Could you check a few things on this model? Use its own coordinates, in mm. A direction names the side the tool comes from. Coordinates: 2 decimals unless noted, no trailing zeros. Loops run counter-clockwise (first coordinate to the right, second up) from the corner with the lowest first, then second, coordinate; pieces in that order, holes last.
1) Will these pins go through, and if not, where does the flat tip stop? P1, Ø8, axis at x = -11.5, z = 19, coming from the -Y side; P2, Ø2, axis at y = -26, z = 18, coming from the +X side; P3, Ø1.5, axis at y = 19, z = 15, coming from the -X side.
2) For faces 1 (the face through (-5.9, -37.15, 12.56)), 2 (the face through (4.52, -97.52, -4.35)), which set-ups out of +Z, -Z, +X, -X, +Y, -Y let a thin tool reach every point of the face, with its end or its side?
3) Imagine slicing it at A-A on y = -52. Please give me the cut outline in (x, z).
4) Thinking about a two-plate mould opening in Y: for faces 3 (the face through (-4.764, 5.484, 13.786)), 4 (the face through (-9.19, -104.525, 17.902)), 5 (the face through (-2, 83.25, 6.23)), 6 (the face through (1.7, -26.055, 0.225)), which applies, released by +Y, released by -Y, zero draft, split by the parting line, or undercut?
5) If I drill on line 1 along X through (y, z) = (19, 5.5); line 2 along Y through (x, z) = (-1, 5); line 3 along Z through (x, y) = (-7, -86), over which ranges is the centre line in solid material (lowest first)?
6) Imagine slicing it at B-B on z = 22. Please give me the cut outline in (x, y), plus the area to 3 significant figures.
Autodesk Inventor part; units mm, degrees
ref_plane "Work Plane2" through (0, -19.1092, 0) normal (0.8514, 0, 0.5245) x (0.513, -0.2079, -0.8328)
ref_plane "YZ Plane" through (0, 0, 0) normal (1, 0, 0) x (0, 1, 0)
ref_plane "XZ Plane" through (0, 0, 0) normal (0, 1, 0) x (-1, 0, 0)
ref_plane "Work Plane2" through (0, -19.1092, 0) normal (0.8514, 0, 0.5245) x (0.513, -0.2079, -0.8328)
ref_plane "Work Plane1" through (99.2081, 0, -373.4906) normal (0.8514, 0, 0.5245) x (0.513, -0.2079, -0.8328)
sketch "Sketch1" plane through (0, -19.1092, 0) normal (0.8514, 0, 0.5245) x (0.513, -0.2079, -0.8328)
  line L0 (-64.4031, -17.2568) -> (64.4031, 17.2568) construction
  line L1 (57.9081, 47.8134) -> (-73.8002, 26.9529) construction
  line L2 (-73.8887, 27.5118) -> (57.8196, 48.3724) construction
  line L3 (54.5542, 79.4406) -> (-78.6131, 72.4616) construction
  line L4 (-78.6427, 73.0267) -> (54.5245, 80.0057) construction
  line L5 (54.5245, 111.2451) -> (-78.6427, 118.2241) construction
  line L6 (64.5496, 16.7101) -> (-64.2566, -17.8034) construction
  line L7 (-50.2899, -60.7886) -> (74.2031, -13.0002) construction
  line L8 (-31.7037, -102.6067) -> (87.112, -42.0671) construction
  line L9 (74.4059, -13.5286) -> (-50.0871, -61.3169) construction
  line L10 (0.1465, -0.5466) -> (11.9566, -36.8944)
  line L11 (12.1594, -37.4227) -> (11.9566, -36.8944)
  line L12 (0, 0) -> (0.1465, -0.5466)
  line L13 (0, 0) -> (-7.946, 37.3832)
  line L14 (-8.0346, 37.9421) -> (-7.946, 37.3832)
  line L15 (12.1594, -37.4227) -> (27.7042, -72.3369)
  line L16 (-8.0346, 37.9421) -> (-12.0295, 75.9511)
  line L17 (-12.0591, 76.5162) -> (-12.0591, 114.7346)
  line L18 (-12.0591, 114.7346) -> (-51.1841, 106.4183)
  line L19 (-51.1841, 106.4183) -> (-11.4208, -80.6532)
  line L20 (-11.4208, -80.6532) -> (27.7042, -72.3369)
  line L21 (-12.0591, 76.5162) -> (-12.0295, 75.9511)
  line L22 (-5.7011, 18.3243) -> (-6.9685, 24.2871)
  line L23 (-5.7011, 18.3243) -> (-4.4336, 12.3615)
  line L24 (-6.9685, 24.2871) -> (-15.7828, 22.4135)
  line L25 (-13.2479, 10.488) -> (-4.4336, 12.3615)
  line L26 (-13.8552, 13.3451) -> (-15.1754, 19.5564)
  line L27 (-15.1754, 19.5564) -> (-15.7828, 22.4135)
  line L28 (-13.8552, 13.3451) -> (-13.2479, 10.488)
  line L29 (-23.1083, 11.3783) -> (-24.4286, 17.5896)
  line L30 (-24.4286, 17.5896) -> (-15.1754, 19.5564)
  line L31 (-13.8552, 13.3451) -> (-23.1083, 11.3783)
  line L32 (2.7351, -66.0118) -> (0.1524, -60.2107)
  line L33 (-12.2145, -27.9939) -> (-14.1768, -21.9547)
  line L34 (-29.827, 51.6736) -> (-30.4907, 57.9888)
  line L35 (-32.2968, 92.4504) -> (-32.2968, 98.8004)
  line L36 (-3.2177, -25.0707) -> (-5.1799, -19.0315)
  line L37 (11.3771, -62.1641) -> (8.7944, -56.3631)
  line L38 (-20.4189, 52.6624) -> (-21.0827, 58.9776)
  line L39 (-22.8369, 92.4504) -> (-22.8369, 98.8004)
  line L40 (2.7351, -66.0118) -> (11.3771, -62.1641)
  line L41 (8.7944, -56.3631) -> (0.1524, -60.2107)
  line L42 (-3.2177, -25.0707) -> (-12.2145, -27.9939)
  line L43 (-14.1768, -21.9547) -> (-5.1799, -19.0315)
  line L44 (-29.827, 51.6736) -> (-20.4189, 52.6624)
  line L45 (-21.0827, 58.9776) -> (-30.4907, 57.9888)
  line L46 (-32.2968, 92.4504) -> (-22.8369, 92.4504)
  line L47 (-22.8369, 98.8004) -> (-32.2968, 98.8004)
  line L48 (5.3525, -22.2861) -> (6.2551, -25.0641)
  line L49 (6.2551, -25.0641) -> (-2.315, -27.8487)
  line L50 (-2.315, -27.8487) -> (-3.2177, -25.0707)
  line L51 (3.3902, -16.2468) -> (2.4876, -13.4688)
  line L52 (2.4876, -13.4688) -> (-6.0826, -16.2534)
  line L53 (-6.0826, -16.2534) -> (-5.1799, -19.0315)
  line L54 (19.6093, -58.4989) -> (20.7973, -61.1674)
  line L55 (20.7973, -61.1674) -> (12.5652, -64.8325)
  line L56 (8.7944, -56.3631) -> (7.6063, -53.6946)
  line L57 (7.6063, -53.6946) -> (15.8384, -50.0294)
  line L58 (15.8384, -50.0294) -> (17.0265, -52.6979)
  line L59 (12.5652, -64.8325) -> (11.3771, -62.1641)
  line L60 (-11.4571, 53.6043) -> (-11.1518, 50.6993)
  line L61 (-11.1518, 50.6993) -> (-20.1136, 49.7574)
  line L62 (-20.1136, 49.7574) -> (-20.4189, 52.6624)
  line L63 (-12.1209, 59.9195) -> (-12.4262, 62.8245)
  line L64 (-12.4262, 62.8245) -> (-21.388, 61.8826)
  line L65 (-21.388, 61.8826) -> (-21.0827, 58.9776)
  line L66 (-13.8257, 92.4504) -> (-13.8257, 89.5294)
  line L67 (-13.8257, 89.5294) -> (-22.8369, 89.5294)
  line L68 (-22.8369, 89.5294) -> (-22.8369, 92.4504)
  line L69 (-22.8369, 98.8004) -> (-22.8369, 101.7214)
  line L70 (-22.8369, 101.7214) -> (-13.8257, 101.7214)
  line L71 (-13.8257, 101.7214) -> (-13.8257, 98.8004)
  line L72 (8.7177, -21.1926) -> (5.3525, -22.2861)
  line L73 (6.7555, -15.1534) -> (3.3902, -16.2468)
  line L74 (-10.2873, 92.4504) -> (-13.8257, 92.4504)
  line L75 (-10.2873, 98.8004) -> (-13.8257, 98.8004)
  line L76 (-7.938, 53.9742) -> (-11.4571, 53.6043)
  line L77 (-8.6018, 60.2894) -> (-12.1209, 59.9195)
  line L78 (22.8418, -57.0597) -> (19.6093, -58.4989)
  line L79 (20.259, -51.2587) -> (17.0265, -52.6979)
  line L80 (-13.8257, 101.7214) -> (-12.0591, 101.7214)
  line L81 (-13.8257, 89.5294) -> (-12.0591, 89.5294)
  line L82 (-12.4262, 62.8245) -> (-10.6692, 63.0092)
  line L83 (-11.1518, 50.6993) -> (-9.3948, 50.884)
  line L84 (-6.9685, 24.2871) -> (-5.2404, 24.6544)
  line L85 (-4.4336, 12.3615) -> (-2.7056, 12.7288)
  line L86 (2.4876, -13.4688) -> (4.1678, -12.9229)
  line L87 (6.2551, -25.0641) -> (7.9353, -24.5182)
  line L88 (15.8384, -50.0294) -> (17.4523, -49.3109)
  line L89 (20.7973, -61.1674) -> (22.4113, -60.4488)
  line L90 (-1.5798, 15.9543) -> (-5.041, 15.2187)
  line L91 (-5.041, 15.2187) -> (-6.3612, 21.4299)
  line L92 (-2.9001, 22.1656) -> (-6.3612, 21.4299)
  line L93 (-1.5798, 15.9543) -> (-2.9001, 22.1656)
  line L94 (-13.8257, 92.4504) -> (-13.8257, 98.8004)
  line L95 (-10.2873, 92.4504) -> (-10.2873, 98.8004)
  line L96 (-11.4571, 53.6043) -> (-12.1209, 59.9195)
  line L97 (-7.938, 53.9742) -> (-8.6018, 60.2894)
  line L98 (5.3525, -22.2861) -> (3.3902, -16.2468)
  line L99 (8.7177, -21.1926) -> (6.7555, -15.1534)
  line L100 (19.6093, -58.4989) -> (17.0265, -52.6979)
  line L101 (22.8418, -57.0597) -> (20.259, -51.2587)
  point P0 (-13.8697, 13.4133)
  point P1 (4.3713, -19.2665)
  point P2 (18.3179, -55.5984)
  point P3 (-11.789, 56.7619)
  point P4 (-13.8257, 95.6254)
  dimension "d0" = 27.94
  dimension "d16" = 6.096
  dimension "d17" = 6.096
  dimension "d20" = 6.096
  dimension "d21" = 6.096
  dimension "d22" = 6.096
  dimension "d23" = 6.096
  dimension "d24" = 6.096
  dimension "d25" = 6.096
  dimension "d26" = 6.096
  dimension "d27" = 6.096
extrude "Extrusion1" add sketch "Sketch1" along normal blind 3.175 contours L10 L86 L52 L53 L43 L33 L42 L50 L49 L87 L11 L15 L88 L57 L56 L41 L32 L40 L59 L55 L89 L20 L19 L18 L17 L80 L70 L69 L47 L35 L46 L68 L67 L81 L21 L16 L82 L64 L65 L45 L34 L44 L62 L61 L83 L14 L13 L84 L24 L27 L30 L29 L31 L28 L25 L85 L12
sketch "Sketch3" plane through (0, -19.1092, 0) normal (-0.8514, 0, -0.5245) x (-0.513, 0.2079, 0.8328)
  line L0 (-5.2011, -84.1204) -> (-3.7597, -81.2915)
  line L1 (-16.5169, -78.3547) -> (-15.0754, -75.5258)
  line L2 (-26.3912, -69.7601) -> (32.4461, -99.7392)
  line L3 (11.4208, -80.6532) -> (-27.7042, -72.3369)
  line L4 (-27.7042, -72.3369) -> (-27.8194, -72.5958)
  line L5 (-27.8194, -72.5958) -> (-16.5169, -78.3547)
  line L6 (-5.2011, -84.1204) -> (9.1316, -91.4233)
  line L7 (9.1316, -91.4233) -> (11.4208, -80.6532)
  line L8 (51.1841, 106.4183) -> (11.4208, -80.6532)
  line L9 (-27.7042, -72.3369) -> (-12.1594, -37.4227)
  line L10 (37.5756, 113.1758) -> (37.4095, 116.3465)
  line L11 (24.893, 112.5111) -> (24.7269, 115.6818)
  line L12 (12.2104, 111.8465) -> (78.1546, 115.3025)
  line L13 (37.4095, 116.3465) -> (53.4733, 117.1883)
  line L14 (53.4733, 117.1883) -> (51.1841, 106.4183)
  line L15 (12.0591, 76.5162) -> (12.0591, 114.7346)
  line L16 (12.0591, 114.7346) -> (12.0591, 115.0179)
  line L17 (12.0591, 115.0179) -> (24.7269, 115.6818)
  line L18 (12.0591, 76.5162) -> (12.0591, 114.7346)
  line L19 (12.0591, 114.7346) -> (51.1841, 106.4183)
  point P0 (3.973, 18.6916)
  point P1 (-3.7597, -81.2915)
  point P2 (37.5756, 113.1758)
  point P3 (24.893, 112.5111)
extrude "Extrusion2" add sketch "Sketch3" against normal blind 3.175
equation "\"d17\" = d16"
properties part number "Center Plate" material "Aluminum 6061"
Filled in:
1. P1: stops at y = -106.17
1. P2: stops at x = -6.74
1. P3: stops at x = -9.7
2. face 1: -Z, +X
2. face 2: -Z, +X, -Y
3. outline: (-14.65, 23.79) - (1.8, -2.92) - (4.5, -1.25) - (-11.95, 25.45) - close
4. face 3: zero draft
4. face 4: released by -Y
4. face 5: undercut
4. face 6: undercut
5. line 1: x = -3.39 to 0.34
5. line 2: y = -97.14 to -82.91, -76.42 to -45.52, -33.26 to -6.1, 6.1 to 33.26, 45.52 to 76.42, 82.91 to 97.14
5. line 3: z = 11.36 to 17.42
6. outline: (-13.55, -106.07) - (-9.82, -105.55) - (-9.82, 105.55) - (-13.55, 106.07) - close
6. area: 789 mm2
